Source: CAD feature listing. Evaluate the final solid. Frame: model axes, mm. Coordinates: 2 decimals unless noted, no trailing zeros. Order: outer loops, then holes, each group sorted by start corner. A loop starts at its lowest first (then second) coordinate and runs counter-clockwise, first axis right, second up. Notation, with made-up numbers: (-6, 58.25) -> (-1, 58.25) arc R13 cw to (-1, 81.25) -> close; hole circle Ø9 at (25.5, -11.75). An arc over 180 degrees is marked (long way). Put each result on its own line as item: value.
from build123d import *

# Parameters (mm, degrees)
SKETCH1_W               = 34.925
SKETCH1_H               = 25.4
BOSS_EXTRUDE1_DEPTH     = 2.54
CUT_EXTRUDE3_DEPTH      = 44.259302179
CUT_EXTRUDE3_DEPTH_BACK = 44.259302179
SKETCH2_R               = 1.5
SKETCH5_R               = 1.1303
CUT_EXTRUDE4_DEPTH      = 44.259302179


with BuildPart() as part:
    # Sketch1 → Boss-Extrude1 (new body)
    with BuildSketch(Plane(origin=(0, 0, 0), x_dir=(1, 0, 0), z_dir=(0, 1, 0))):
        with Locations((17.4625, 12.7)):
            Rectangle(SKETCH1_W, SKETCH1_H)
    extrude(amount=BOSS_EXTRUDE1_DEPTH)

    # Sketch2 → Cut-Extrude3 (cut, two sides: drawn at the far end of the back side and taken through both)
    with BuildSketch(Plane(origin=(0, 2.54, 0), x_dir=(1, 0, 0), z_dir=(0, 1, 0)).offset(-CUT_EXTRUDE3_DEPTH_BACK)):
        with Locations(Location((3.81, 19.2, 0), (0, 0, 90))):
            Circle(SKETCH2_R)
        with Locations(Location((3.81, 6.2, 0), (0, 0, 90))):
            Circle(SKETCH2_R)
    extrude(amount=CUT_EXTRUDE3_DEPTH + CUT_EXTRUDE3_DEPTH_BACK, mode=Mode.SUBTRACT)

    # Sketch5 → Cut-Extrude4 (cut, through all)
    with BuildSketch(Plane(origin=(0, 2.54, 0), x_dir=(1, 0, 0), z_dir=(0, 1, 0))):
        with Locations(Location((31.75, 20.32, 0), (0, 0, 270))):
            Circle(SKETCH5_R)
        with Locations(Location((31.75, 5.08, 0), (0, 0, 90))):
            Circle(SKETCH5_R)
    extrude(amount=-CUT_EXTRUDE4_DEPTH, mode=Mode.SUBTRACT)


solid = part.part
1. Cut plane C-C on z = -5.5. Output: boundary loops of the cut face in (x, y) (3 decimals), plus the area to 3 significant figures.
Numbers:
outline: (0, 0) -> (2.483, 0) -> (2.483, 2.54) -> (0, 2.54) -> close; (5.137, 0) -> (30.701, 0) -> (30.701, 2.54) -> (5.137, 2.54) -> close; (32.799, 0) -> (34.925, 0) -> (34.925, 2.54) -> (32.799, 2.54) -> close
area: 76.6 mm2
2. Cut plane A-A on x = 31.75. Output: boundary loops of the cut face in (y, z), plus the area to 3 significant figures.
Numbers:
outline: (0, -25.4) -> (2.54, -25.4) -> (2.54, -21.45) -> (0, -21.45) -> close; (0, -19.19) -> (2.54, -19.19) -> (2.54, -6.21) -> (0, -6.21) -> close; (0, -3.95) -> (2.54, -3.95) -> (2.54, 0) -> (0, 0) -> close
area: 53.0 mm2
3. Pull-direction query (X, two-part tool) for faces 1 (the flat face through (17, 1, -25.4)), 2 (the flat face through (34.925, 1, -13)), 3 (the cylindrical face through (3.36, 1.25, -20.63)); classes: pulls with the +X half, pulls with the -X half, needs draft (parallel to the pull), parting line crosses it, or undercut.
Numbers:
face 1: needs draft
face 2: pulls with the +X half
face 3: undercut
4. Ray query, line 1 along X through (y, z) = (1.25, -6) (3 decimals); line 2 along X through (y, z) = (1.7, -20.32) (3 decimals); line 3 along Z through (x, y) = (32, 1.8). Return the intervals inside material, ascending.
Numbers:
line 1: x = 0 to 2.323, 5.297 to 31.093, 32.407 to 34.925
line 2: x = 0 to 2.812, 4.808 to 30.62, 32.88 to 34.925
line 3: z = -25.4 to -21.42, -19.22 to -6.18, -3.98 to 0
5. Cut plane B-B on y = 1.85. Output: boundary loops of the cut face in (x, z) (3 decimals).
Numbers:
outline: (0, -25.4) -> (34.925, -25.4) -> (34.925, 0) -> (0, 0) -> close; hole circle Ø3 at (3.81, -19.2); hole circle Ø3 at (3.81, -6.2); hole circle Ø2.261 at (31.75, -20.32); hole circle Ø2.261 at (31.75, -5.08)
